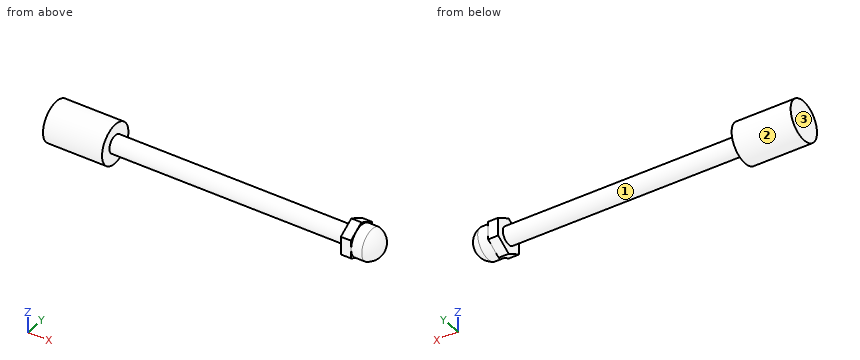
from build123d import *

# Parameters (mm, degrees)
SKETCH8_R           = 3.4
BOSS_EXTRUDE1_DEPTH = 10
SKETCH9_R           = 1.5
BOSS_EXTRUDE2_DEPTH = 40
BOSS_EXTRUDE3_DEPTH = 1.7
SKETCH11_R          = 2.65
BOSS_EXTRUDE4_DEPTH = 1.8
DOME1_FACE_RADIUS   = 2.65
DOME1_HEIGHT        = 2


with BuildPart() as part:
    # Sketch8 → Boss-Extrude1 (new body)
    with BuildSketch(Plane(origin=(0, 0, 0), x_dir=(0, 0, -1), z_dir=(1, 0, 0))):
        Circle(SKETCH8_R)
    extrude(amount=BOSS_EXTRUDE1_DEPTH)

    # Sketch9 → Boss-Extrude2 (add)
    with BuildSketch(Plane(origin=(10, 0, 0), x_dir=(0, 0, -1), z_dir=(1, 0, 0))):
        Circle(SKETCH9_R)
    extrude(amount=BOSS_EXTRUDE2_DEPTH)

    # Sketch10 → Boss-Extrude3 (add)
    with BuildSketch(Plane(origin=(50, 0, 0), x_dir=(0, 0, -1), z_dir=(1, 0, 0))):
        Polygon((-1.558845727, 2.7), (1.558845727, 2.7), (3.117691454, 0), (1.558845727, -2.7), (-1.558845727, -2.7), (-3.117691454, 0), align=None)
    extrude(amount=BOSS_EXTRUDE3_DEPTH)

    # Sketch11 → Boss-Extrude4 (add)
    with BuildSketch(Plane(origin=(51.7, 0, 0), x_dir=(0, 0, -1), z_dir=(1, 0, 0))):
        Circle(SKETCH11_R)
    extrude(amount=BOSS_EXTRUDE4_DEPTH)

    # Dome1: a dome of height H over a round flat face of radius A is a cap of a sphere of radius (A * A + H * H) / (2 * H)
    dome1_r = (DOME1_FACE_RADIUS * DOME1_FACE_RADIUS + DOME1_HEIGHT * DOME1_HEIGHT) / (2 * DOME1_HEIGHT)
    dome1_base = Plane((53.5, 0, 0), z_dir=(1, 0, 0))
    with Locations(dome1_base.offset(DOME1_HEIGHT - dome1_r)):
        dome1_ball = Sphere(dome1_r, mode=Mode.PRIVATE)
    add(split(dome1_ball, bisect_by=dome1_base, keep=Keep.TOP, mode=Mode.PRIVATE))


solid = part.part
The listing builds one solid part. Answer for the finished solid, in the listing's coordinates (mm). Face numbers are marked on the shaded views. Round coordinates to 2 decimals unless told otherwise and drop trailing zeros. Write each loop counter-clockwise with the first axis right and the second up, starting at its lowest first coordinate (ties: lowest second). Pieces come first, ordered by that corner, then holes. Notation, with made-up numbers: M -38,-34 L 12,-34 A15 cw 12,-5 Z; hole C 75,0 d6. An arc over 180 degrees is marked long. Write each question's results on one line, items separated by ' | '. Start each with the question number.
(1) The part is cut by section A-A, the plane z = 0. Write down the section's boundary in (x, y), and give its area (3 significant figures).
(2) Each of these flat-tipped pins is pushed along its axis until it touches: P1, Ø2, axis at y = 1, z = 2.5, coming from the +X side; P2, Ø1.5, axis at y = -1, z = 0, coming from the -X side; P3, Ø0.9, axis at x = 51, z = 0, coming from the -Y side; P4, Ø0.5, axis at x = 51, z = 0.5, coming from the +Y side. Where does it stop, or does it pass through?
(3) The part is cut by section B-B, the plane x = 30. Write down the section's boundary in (y, z), and give its area (3 significant figures).
(4) Determine the mould class of the marked faces 1, 2 and 3 for opening direction X: +X half, -X half, draft (parallel to the pull), parting line (faces both ways), or undercut.
(5) The part is cut by section C-C, the plane x = 9.5. Write down the section's boundary in (y, z).
(6) Find the intervals of material crossed by line 1 (X direction, y = 0.5, z = 2.75); line 2 (X direction, y = -2, z = -1.25); line 3 (X direction, y = -1.5, z = 2.75), in increasing order.
Worked answers:
1) outline: M 0,-3.4 L 10,-3.4 L 10,-1.5 L 50,-1.5 L 50,-2.7 L 51.7,-2.7 L 51.7,-2.65 L 53.5,-2.65 A2.76 ccw 53.5,2.65 L 51.7,2.65 L 51.7,2.7 L 50,2.7 L 50,1.5 L 10,1.5 L 10,3.4 L 0,3.4 Z | area: 215 mm²
2) P1: stops at x = 54.92 | P2: stops at x = 0 | P3: stops at y = -2.7 | P4: stops at y = 2.7
3) outline: C 0,0 d3 | area: 7.07 mm²
4) face 1: undercut | face 2: draft | face 3: -X half
5) outline: C 0,0 d6.8
6) line 1: x = 0 to 10, 50 to 51.7 | line 2: x = 0 to 10, 50 to 54.17 | line 3: x = 0 to 10
